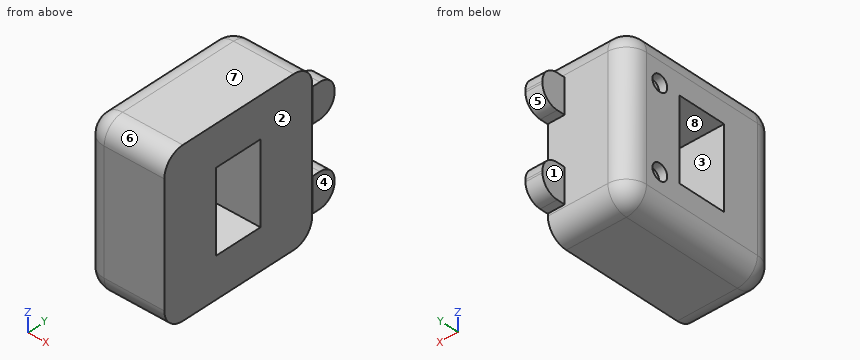
Autodesk Inventor part; units mm, degrees
ref_plane "YZ Plane" through (0, 0, 0) normal (1, 0, 0) x (0, 1, 0)
ref_plane "XZ Plane" through (0, 0, 0) normal (0, 1, 0) x (-1, 0, 0)
ref_plane "XY Plane" through (0, 0, 0) normal (0, 0, 1) x (1, 0, 0)
sketch "Sketch1" plane through (0, 0, 0) normal (0, 0, 1) x (1, 0, 0)
  line L0 (6.35, -12.6955) -> (-3.175, -12.6955)
  line L1 (-6.35, -9.5205) -> (-6.35, 9.5205)
  line L2 (-3.175, 12.6955) -> (6.35, 12.6955)
  line L3 (6.35, 12.6955) -> (6.35, -12.6955)
  line L4 (6.35, -12.6955) -> (-6.35, 12.6955) construction
  line L5 (-6.35, -12.6955) -> (6.35, 12.6955) construction
  arc A0 (-3.175, 12.6955) -> (-6.35, 9.5205) centre (-3.175, 9.5205) ccw
  arc A1 (-6.35, -9.5205) -> (-3.175, -12.6955) centre (-3.175, -9.5205) ccw
  point P0 (0, 0)
  dimension "d0" = 12.7
  dimension "d1" = 3.175
extrude "Extrusion1" add sketch "Sketch1" along normal blind 25.4
fillet "Fillet1" radius 3.175 10 edges at (-6.35, 0, 25.4) (-5.4201, -11.7656, 25.4) (1.5875, -12.6955, 25.4) (1.5875, 12.6955, 25.4) (-5.4201, 11.7656, 25.4) (-5.4201, 11.7656, 0) (1.5875, 12.6955, 0) (-5.4201, -11.7656, 0) (1.5875, -12.6955, 0) (-6.35, 0, 0)
sketch "Sketch2" plane through (-3.175, 12.6955, 3.175) normal (0, 1, 0) x (1, 0, 0)
  circle A0 centre (2.6716, -16.206) radius 2.54
  line L0 (0, 0) -> (0, -19.05)
  line L1 (9.525, 0) -> (9.525, -19.05)
  circle A1 centre (2.6716, -2.844) radius 2.54
  point P0 (3.175, 3.175)
  dimension "d5" = 5.08
extrude "Extrusion2" add sketch "Sketch2" along normal blind 12.7
sketch "Sketch3" plane through (-6.35, -9.5205, 3.175) normal (-1, 0, 0) x (0, 0, 1)
  line L0 (4.445, 6.9805) -> (14.605, 12.0605) construction
  line L1 (14.605, 6.9805) -> (4.445, 12.0605) construction
  line L2 (3.175, 5.7105) -> (3.175, 13.3305)
  line L3 (15.875, 13.3305) -> (15.875, 5.7105)
  line L4 (15.875, 5.0755) -> (3.175, 13.9655) construction
  line L5 (3.175, 5.0755) -> (15.875, 13.9655) construction
  line L6 (3.175, 13.3305) -> (15.875, 13.3305)
  line L7 (15.875, 13.3305) -> (15.875, 5.7105)
  line L8 (15.875, 5.7105) -> (3.175, 5.7105)
  line L9 (3.175, 5.7105) -> (3.175, 13.3305)
  line L10 (3.175, 13.3305) -> (15.875, 5.7105) construction
  line L11 (15.875, 13.3305) -> (3.175, 5.7105) construction
  point P0 (-3.175, 9.5205)
  point P1 (9.525, 9.5205)
  point P2 (15.875, 12.0605)
  point P3 (15.875, 6.9805)
  dimension "d25" = 7.62
extrude "Extrusion3" cut sketch "Sketch3" against normal blind 12.7
sketch "Sketch4" plane through (-0.5034, 25.3955, 19.381) normal (0, 1, 0) x (1, 0, 0)
  line L0 (-9.3616, 22.1264) -> (11.0198, 22.1264)
  line L1 (11.0198, 22.1264) -> (11.0198, -9.2368)
  line L2 (11.0198, -9.2368) -> (-9.3616, -9.2368)
  line L3 (-9.3616, -9.2368) -> (-9.3616, 22.1264)
  point P0 (0.5034, 19.381)
extrude "Extrusion4" cut sketch "Sketch4" against normal blind 12.7
sketch "Sketch5" plane through (-3.175, 12.6955, 3.175) normal (0, 1, 0) x (1, 0, 0)
  line L0 (6.852, -0.3615) -> (9.5509, -0.3615)
  line L1 (9.5509, -0.3615) -> (9.5509, -5.7593)
  line L2 (9.5509, -5.7593) -> (6.852, -5.7593)
  line L3 (6.852, -5.7593) -> (6.852, -0.3615)
  line L4 (6.852, -0.3615) -> (9.5509, -5.7593) construction
  line L5 (9.5509, -0.3615) -> (6.852, -5.7593) construction
  line L6 (0, 0) -> (0, -19.05)
  line L7 (9.525, 0) -> (9.525, -19.05)
  line L8 (6.852, -18.6885) -> (9.5509, -18.6885)
  line L9 (9.5509, -18.6885) -> (9.5509, -13.2907)
  line L10 (9.5509, -13.2907) -> (6.852, -13.2907)
  line L11 (6.852, -13.2907) -> (6.852, -18.6885)
  line L12 (6.852, -18.6885) -> (9.5509, -13.2907) construction
  line L13 (9.5509, -18.6885) -> (6.852, -13.2907) construction
  point P0 (3.175, 3.175)
  point P1 (8.2015, -3.0604)
  point P2 (8.2015, -15.9896)
extrude "Extrusion5" add sketch "Sketch5" along normal blind 3.81
fillet "Fillet2" radius 2.54 4 edges at (5.0265, 16.5055, 8.9343) (5.0265, 16.5055, 3.5365) (5.0265, 16.5055, 16.4657) (5.0265, 16.5055, 21.8635)
sketch "Sketch7" plane through (-6.35, -9.5205, 3.175) normal (-1, 0, 0) x (0, 0, 1)
  circle A0 centre (3.0142, 16.7412) radius 1.27
  circle A1 centre (15.8269, 16.7412) radius 1.27
  point P0 (-3.175, 9.5205)
  dimension "d26" = 2.54
  dimension "d27" = 2.54
extrude "Extrusion7" cut sketch "Sketch7" against normal blind 1.27
properties part number "pig_face"
Verification items for the finished model (mm, model axes). Face numbers are marked on the shaded views. A direction names the side the tool comes from. Coordinates: 2 decimals unless noted, no trailing zeros. Order: outer loops, then holes, each group sorted by start corner. A loop starts at its lowest first (then second) coordinate and runs counter-clockwise, first axis right, second up. Notation, with made-up numbers: (1.25, 54) -> (27.25, 54) arc R18 cw to (27.25, 58) -> close; hole circle Ø2 at (40, 2). An arc over 180 degrees is marked (long way). Put each result on its own line as item: value. Start each with the question number.
1) Material ranges on L1, parallel to Y at x = 0.5, z = 16.5; L2, parallel to X at y = -4.5, z = 11.25; L3, parallel to Y at x = -5, z = 10, recorded low to high.
2) Go/stop test with flat-tipped pins: pin 1 (3 mm diameter, centred on y = 6, z = 21.5, fed in from +X); pin 2 (0.6 mm diameter, centred on x = 5, y = 13.5, fed in from -Z); pin 3 (3 mm diameter, centred on x = 5, z = 21.5, fed in from +Y). Record where each tip stops, or that it passes through.
3) Cross-section at B-B (y = 2.75). Enter the section's corners in (x, z) (3 decimals).
4) Tool access check on the marked faces 1, 2, 3 and 4. Record the directions out of +Z, -Z, +X, -X, +Y, -Y that give a thin tool (end or side, any length) a straight path to the whole face; none if there is none.
5) Release check for a two-part mould opening along Y. For the marked faces 5, 6, 7 and 8 record: pulls with the +Y half, pulls with the -Y half, needs draft (parallel to the pull), parting line crosses it, or undercut.
Geometry check:
1. L1: y = -12.7 to -3.81, 3.81 to 12.7
1. L2: x = -6.35 to 6.35
1. L3: y = -12.12 to -3.81, 3.81 to 12.12
2. pin 1: stops at x = 6.35
2. pin 2: stops at z = 3.54
2. pin 3: stops at y = 16.41
3. outline: (-6.35, 3.175) arc R3.175 ccw to (-3.175, 0) -> (6.35, 0) -> (6.35, 6.35) -> (-6.35, 6.35) -> close; (-6.35, 19.05) -> (6.35, 19.05) -> (6.35, 25.4) -> (-3.175, 25.4) arc R3.175 ccw to (-6.35, 22.225) -> close
4. face 1: +Z, -Z, -X, +Y
4. face 2: +Z, -Z, +X, -Y
4. face 3: +X, -X
4. face 4: +Z, -Z, +X, +Y, -Y
5. face 5: pulls with the +Y half
5. face 6: pulls with the -Y half
5. face 7: needs draft
5. face 8: undercut
